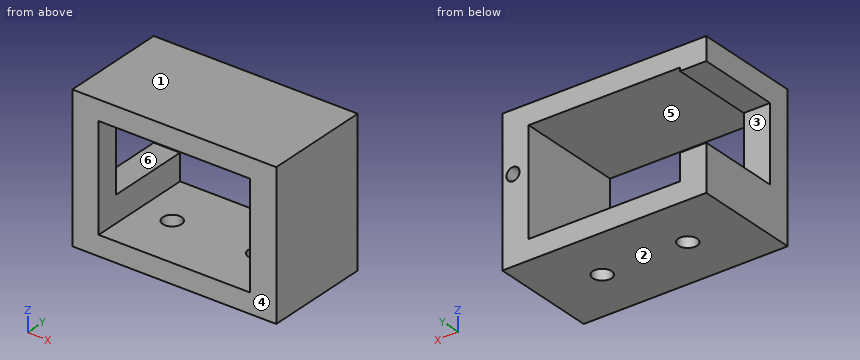
```python
from build123d import *

# Parameters (mm, degrees)
SKETCH2_W           = 31
SKETCH2_H           = 21.9
BOSS_EXTRUDE1_DEPTH = 16.25
SKETCH3_W           = 23
SKETCH3_H           = 15.9
CUT_EXTRUDE1_DEPTH  = 25.984295067
SKETCH6_R           = 1.4224
CUT_EXTRUDE3_DEPTH  = 10
SKETCH7_W           = 11.4
SKETCH7_H           = 9.25
CUT_EXTRUDE4_DEPTH  = 10
SKETCH9_R           = 1
CUT_EXTRUDE5_DEPTH  = 10
SKETCH12_W          = 11.4
SKETCH12_H          = 3.5
CUT_EXTRUDE8_DEPTH  = 4


with BuildPart() as part:
    # Sketch2 → Boss-Extrude1 (new body)
    with BuildSketch(Plane(origin=(0, 0, 0), x_dir=(1, 0, 0), z_dir=(0, 1, 0))):
        Rectangle(SKETCH2_W, SKETCH2_H)
    extrude(amount=BOSS_EXTRUDE1_DEPTH)

    # Sketch3 → Cut-Extrude1 (cut, through all)
    with BuildSketch(Plane(origin=(0, 16.25, 0), x_dir=(1, 0, 0), z_dir=(0, 1, 0))):
        Rectangle(SKETCH3_W, SKETCH3_H)
    extrude(amount=-CUT_EXTRUDE1_DEPTH, mode=Mode.SUBTRACT)

    # Sketch6 → Cut-Extrude3 (cut)
    with BuildSketch(Plane(origin=(0, 0, -10.95), x_dir=(-1, 0, 0), z_dir=(0, 0, -1))):
        with Locations((-6.5, 8.125)):
            Circle(SKETCH6_R)
        with Locations((6.5, 8.125)):
            Circle(SKETCH6_R)
    extrude(amount=-CUT_EXTRUDE3_DEPTH, mode=Mode.SUBTRACT)

    # Sketch7 → Cut-Extrude4 (cut)
    with BuildSketch(Plane.ZY.offset(15.5)):
        with Locations((1.75, 8.125)):
            Rectangle(SKETCH7_W, SKETCH7_H)
    extrude(amount=-CUT_EXTRUDE4_DEPTH, mode=Mode.SUBTRACT)

    # Sketch9 → Cut-Extrude5 (cut)
    with BuildSketch(Plane(origin=(0, 16.25, 0), x_dir=(1, 0, 0), z_dir=(0, 1, 0))):
        with Locations(Location((-13.37, -1.95, 0), (0, 0, 270))):
            Circle(SKETCH9_R)
        with Locations(Location((13.87, -1.95, 0), (0, 0, 270))):
            Circle(SKETCH9_R)
    extrude(amount=-CUT_EXTRUDE5_DEPTH, mode=Mode.SUBTRACT)

    # Sketch12 → Cut-Extrude8 (cut)
    with BuildSketch(Plane.ZY.offset(15.5)):
        with Locations((1.75, 14.5)):
            Rectangle(SKETCH12_W, SKETCH12_H)
    extrude(amount=-CUT_EXTRUDE8_DEPTH, mode=Mode.SUBTRACT)


solid = part.part
```
Geometry: final body of the model. Coordinates: model frame, mm. Face numbers are marked on the shaded views. A direction names the side the tool comes from. Give positions to 0.01 mm unless a question says otherwise; leave off trailing zeros. Order: outer loops, then holes, each group sorted by start corner. A loop starts at its lowest first (then second) coordinate and runs counter-clockwise, first axis right, second up. Notation, with made-up numbers: (-0.5, 28) -> (20.5, 28) arc R29 ccw to (20.5, 65) -> close; hole circle Ø3 at (43, 4.25). An arc over 180 degrees is marked (long way). Write each question's results on one line, items separated by ' | '. Start each with the question number.
1) Line query: line 1 (X direction, y = 14.25, z = 1.95); line 2 (Z direction, x = -2.5, y = 11.5); line 3 (Y direction, x = 6.5, z = -9.25). Output: solid intervals per line, ascending. Write a range as from..to.
2) Set-up query: the marked faces 4, 5 and 6. Return all of +Z, -Z, +X, -X, +Y, -Y with unobstructed straight access to the full face (end or side cutting, diameter ignored); none if empty.
3) Draft query along Z for the marked faces 1, 2 and 3. Return one class per face: pulls with the +Z half, pulls with the -Z half, needs draft (parallel to the pull), parting line crosses it, or undercut.
4) Section C-C (x = 3). Return loops of the section in (y, z), then the cut area to 3 significant figures.
5) Section A-A (x = 6.5). Return loops of the section in (y, z), then the cut area to 3 significant figures.
6) Section D-D (x = 13.87). Return loops of the section in (y, z), then the cut area to 3 significant figures.
7) Section B-B (y = 2). Return loops of the section in (x, z), then the cut area to 3 significant figures.
8) First-contact query: pin 1 (3 mm diameter, centred on x = -13, z = -0.5, fed in from +Y). Flat tip, straight axial feed; report the tip coordinate or a pass-through.
Calculated:
1) line 1: 11.5..12.87, 14.87..15.5 | line 2: -10.95..-7.95, 7.95..10.95 | line 3: 0..6.7, 9.55..16.25
2) face 4: +Z, -Z, +X, -X, -Y | face 5: +Y, -Y | face 6: -X, +Y
3) face 1: pulls with the +Z half | face 2: pulls with the -Z half | face 3: undercut
4) outline: (0, -10.95) -> (16.25, -10.95) -> (16.25, -7.95) -> (0, -7.95) -> close; (0, 7.95) -> (16.25, 7.95) -> (16.25, 10.95) -> (0, 10.95) -> close | area: 97.5 mm2
5) outline: (0, -10.95) -> (6.7, -10.95) -> (6.7, -7.95) -> (0, -7.95) -> close; (0, 7.95) -> (16.25, 7.95) -> (16.25, 10.95) -> (0, 10.95) -> close; (9.55, -10.95) -> (16.25, -10.95) -> (16.25, -7.95) -> (9.55, -7.95) -> close | area: 89.0 mm2
6) outline: (0, -10.95) -> (16.25, -10.95) -> (16.25, 0.95) -> (6.25, 0.95) -> (6.25, 2.95) -> (16.25, 2.95) -> (16.25, 10.95) -> (0, 10.95) -> close | area: 336 mm2
7) outline: (-15.5, -10.95) -> (15.5, -10.95) -> (15.5, 10.95) -> (-15.5, 10.95) -> close; hole (-11.5, -7.95) -> (11.5, -7.95) -> (11.5, 7.95) -> (-11.5, 7.95) -> close | area: 313 mm2
8) pin 1: y = 3.5
